from build123d import *

# Parameters (mm, degrees)
F0_W     = 25.4
F0_H     = 25.4
F0_W_2   = 50.8
F1_DEPTH = 25.4
F2_DEPTH = 28.956


with BuildPart() as f1:
    # F0 (on Front) → F1 (new body)
    with BuildSketch(Plane.XZ):
        with Locations((-28.554517, -9.791291)):
            Rectangle(F0_W, F0_H)
        with Locations((9.545483, -9.791291)):
            Rectangle(F0_W_2, F0_H)
        with Locations((47.645483, -9.791291)):
            Rectangle(F0_W, F0_H)
        Polygon((-41.254517, 66.408709), (-41.254517, 2.908709), (-15.854517, 2.908709), (34.945483, 2.908709), (60.345483, 2.908709), (60.345483, 66.408709), (34.945483, 94.806772), (34.945483, 44.006772), (-15.854517, 44.006772), (-15.854517, 94.806772), align=None)
    extrude(amount=F1_DEPTH)

    # F1_face (on face) → F2 (join)
    with BuildSketch(Plane(origin=(9.545483, -25.4, 22.080837), x_dir=(1, 0, 0), z_dir=(0, -1, 0))):
        Polygon((-50.8, -44.572128), (50.8, -44.572128), (50.8, 44.327872), (25.4, 72.725935), (25.4, 21.925935), (-25.4, 21.925935), (-25.4, 72.725935), (-50.8, 44.327872), align=None)
    extrude(amount=F2_DEPTH)


solid = f1.part
Source: CAD feature listing. Evaluate the final solid. Frame: model axes, mm. A direction names the side the tool comes from. Give positions to 0.01 mm unless a question says otherwise; leave off trailing zeros. Write each loop counter-clockwise with the first axis right and the second up, starting at its lowest first coordinate (ties: lowest second). Pieces come first, ordered by that corner, then holes. Notation, with made-up numbers: M -27.5,-6 L -0.5,-6 A36 cw -0.5,31 Z; hole C 70.25,82 d10. An arc over 180 degrees is marked long. Answer as a JSON object with one key per item and string values.
Q1. Cut plane A-A, the plane z = 61. Return the cut outline in (x, y).
Geometry check:
{"outline": "M -41.25,-54.36 L -15.85,-54.36 L -15.85,0 L -41.25,0 Z; M 34.95,-54.36 L 60.35,-54.36 L 60.35,0 L 34.95,0 Z"}
Q2. Contact query for flat-ended pins moving along their axis: P1, Ø15, axis at y = -19.5, z = 78.5, coming from the -X side; P2, Ø10, axis at x = 22, y = -47.5, coming from the +Z side; P3, Ø8, axis at x = -18.5, y = -8, coming from the +Z side. Output: stop coordinate, or through.
Geometry check:
{"P1": "stops at x = -37.15", "P2": "stops at z = 44.01", "P3": "stops at z = 94.81"}
Q3. Cut plane B-B, the plane y = -24.5. Return the cut outline in (x, z).
Geometry check:
{"outline": "M -41.25,-22.49 L 60.35,-22.49 L 60.35,66.41 L 34.95,94.81 L 34.95,44.01 L -15.85,44.01 L -15.85,94.81 L -41.25,66.41 Z"}
Q4. Ray query, line 1 along X through (y, z) = (-36.5, 60); line 2 along Z through (x, y) = (-9, -28); line 3 along X through (y, z) = (-36.5, 90). Return the intervals inside material, ascending.
Geometry check:
{"line 1": "x = -41.25 to -15.85, 34.95 to 60.35", "line 2": "z = -22.49 to 44.01", "line 3": "x = -20.15 to -15.85, 34.95 to 39.24"}
Q5. Mould query, pull axis X, two halves, no side actions, for faces 1 (the face through (9, 0, 24)), 2 (the face through (-28.377, -26.798, 80.807)), 3 (the face through (10, -27, 44.007)). Classes: +X half, -X half, draft (parallel to the pull), parting line (faces both ways), or undercut.
Geometry check:
{"face 1": "draft", "face 2": "-X half", "face 3": "undercut"}
Q6. Access query for faces 4 (the face through (34.945, -27, 70)), 5 (the face through (60.345, -27, 21)). Directions: +Z, -Z, +X, -X, +Y, -Y. A direction counts if a zero-diameter tool reaches every point of the face in a straight line with its end or side. Return the directions, or none.
Geometry check:
{"face 4": "+Z, +Y, -Y", "face 5": "+Z, -Z, +X, +Y, -Y"}
Q7. Cut plane C-C, the plane x = 39. Return the cut outline in (y, z), then the cut area to 3 significant figures.
Geometry check:
{"outline": "M -54.36,-22.49 L 0,-22.49 L 0,90.27 L -54.36,90.27 Z", "area": "6,130 mm^2"}
Q8. Cut plane D-D, the plane z = 74. Return the cut outline in (x, y).
Geometry check:
{"outline": "M -34.46,-54.36 L -15.85,-54.36 L -15.85,0 L -34.46,0 Z; M 34.95,-54.36 L 53.56,-54.36 L 53.56,0 L 34.95,0 Z"}
